The model under review builds one solid part; all positions refer to its coordinate system, in mm. A direction names the side the tool comes from. Coordinates: 2 decimals unless noted, no trailing zeros. Write each loop counter-clockwise with the first axis right and the second up, starting at its lowest first coordinate (ties: lowest second). Pieces come first, ordered by that corner, then holes.
1) Add section C-C, the plane x = 2.5. State the section outline as (y, z) points.
2) Add section B-B, the plane z = 40. State the section outline as (x, y) points.
3) For P1, Ø0.6, axis at y = -29.5, z = 53.5, coming from the +X side; P2, Ø10, axis at y = 19, z = 23.5, coming from the +X side; P3, Ø0.6, axis at x = 7, z = 53.5, coming from the +Y side, all flat-tipped, find the tip position at first contact; note any pin that passes through.
4) Mouldability with a two-part tool opening along Y and no side actions: class faces 1 (the cylindrical face through (27.3, 0.2, 77.5)), 2 (the flat face through (-6.705, 9, 45)), 3 (the cylindrical face through (41, -29, 73)), 4 (the flat face through (19.34, -34, 40)) as released by +Y, released by -Y, zero draft, split by the parting line, or undercut.
5) Add section A-A, the plane y = 0. State the section outline as (x, z) points, then the cut area to 3 significant figures.
6) Machinability: for faces 5 (the flat face through (6, -30, 67)), 6 (the flat face through (34.9, -28, 53.3)), 7 (the cylindrical face through (-7.21, 2.6, 59.83)), 8 (the flat face through (34, -34, 27)), 9 (the flat face through (-4, 40, 43)), which of the approach directions +Z, -Z, +X, -X, +Y, -Y give a long, thin tool a straight path to every point of the face, cutting with its end or side? Answer none if there is none.
7) For line 1 (Z direction, x = -4.7, y = 0); line 2 (Z direction, x = 29.5, y = 25); line 3 (X direction, y = 10.5, z = 14), list the stretches that pass through material, from the lowest coordinate up.
from build123d import *

# Parameters (mm, degrees)
SKETCH1_R           = 4.9999999999999964
BOSS_EXTRUDE1_DEPTH = 5
BOSS_EXTRUDE2_DEPTH = 70
BOSS_EXTRUDE3_DEPTH = 70
CUT_EXTRUDE1_DEPTH  = 5
SKETCH6_R           = 20.000000000000004
CUT_EXTRUDE2_DEPTH  = 1
CUT_EXTRUDE3_DEPTH  = 19.000000000000004
BOSS_EXTRUDE4_DEPTH = 1.9999999999999896
FILLET1_R           = 5
CUT_EXTRUDE4_DEPTH  = 27.00000000000001
BOSS_EXTRUDE5_DEPTH = 2
BOSS_EXTRUDE6_DEPTH = 2


with BuildPart() as part:
    # Sketch1 → Boss-Extrude1 (new body)
    with BuildSketch(Plane.XY):
        with BuildLine():
            Line((-7.704615384615421, -40.00000000000001), (32.295384615384584, -40.00000000000001))
            ThreePointArc((32.295384615384584, -40.00000000000001), (72.29538461538459, 0), (32.29538461538458, 39.99999999999999))
            Line((32.29538461538458, 39.99999999999999), (-7.7046153846154315, 39.99999999999999))
            Line((-7.7046153846154315, 39.99999999999999), (-7.704615384615421, -40.00000000000001))
        make_face()
        with Locations((32.295384615384584, 0)):
            Circle(SKETCH1_R, mode=Mode.SUBTRACT)
    boss_extrude1 = extrude(amount=BOSS_EXTRUDE1_DEPTH)

    # Sketch2 → Boss-Extrude2 (add)
    with BuildSketch(Plane.XY.offset(5)):
        Polygon((-7.7046153846154315, 39.99999999999999), (-2.70461538461543, 39.99999999999999), (-2.7046153846154235, -40.00000000000001), (-7.704615384615421, -40.00000000000001), align=None)
    extrude(amount=BOSS_EXTRUDE2_DEPTH)

    # Mirror1: Boss-Extrude1 across plane
    add(boss_extrude1.mirror(Plane.XY.offset(40)))

    # Sketch4 → Boss-Extrude3 (add)
    with BuildSketch(Plane.XY.offset(5)):
        with BuildLine():
            Line((-2.7046153846154266, -40.00000000000001), (-2.7046153846154266, -30.000000000000007))
            Line((-2.7046153846154266, -30.000000000000007), (43.497251593214216, -30.000000000000007))
            Line((43.497251593214216, -30.000000000000007), (58.7528977260305, -30.000000000000007))
            ThreePointArc((58.7528977260305, -30.000000000000007), (46.43752023911554, -37.41657386773942), (32.295384615384584, -40.00000000000001))
            Line((32.295384615384584, -40.00000000000001), (-2.7046153846154266, -40.00000000000001))
        make_face()
    extrude(amount=BOSS_EXTRUDE3_DEPTH)

    # Sketch5 → Cut-Extrude1 (cut)
    with BuildSketch(Plane.ZY.offset(7.704615384615426)):
        with BuildLine():
            ThreePointArc((50.00000000000001, -1.388e-14), (43.82683432365097, 9.238795325112829), (32.92893218813463, 7.071067811865561))
            Line((32.92893218813452, 7.0710678118654755), (47.071067811865476, -7.071067811865483))
            ThreePointArc((47.0710678118656, -7.0710678118653725), (49.2387953251129, -3.826834323650836), (50.00000000000001, -1.633e-14))
        make_face()
        with BuildLine():
            Line((47.071067811865476, -7.071067811865483), (32.92893218813452, 7.0710678118654755))
            ThreePointArc((32.92893218813463, 7.071067811865561), (32.92893218813454, -7.071067811865502), (47.0710678118656, -7.0710678118653725))
        make_face()
    extrude(amount=-CUT_EXTRUDE1_DEPTH, mode=Mode.SUBTRACT)

    # Sketch6 → Cut-Extrude2 (cut)
    with BuildSketch(Plane.ZY.offset(7.704615384615426)):
        with Locations(Location((40.00000000000001, -1.388e-14, 0), (0, 0, 270))):
            Circle(SKETCH6_R)
    extrude(amount=-CUT_EXTRUDE2_DEPTH, mode=Mode.SUBTRACT)

    # Sketch7 → Cut-Extrude3 (cut)
    with BuildSketch(Plane(origin=(0, -30.000000000000007, 0), x_dir=(1, 0, 0), z_dir=(0, 1, 0))):
        Polygon((58.7528977260305, -53.00000000000001), (58.7528977260305, -40.00000000000001), (58.7528977260305, -27.000000000000004), (19.339689979409883, -27.000000000000007), (19.339689979409883, -53.00000000000001), align=None)
    extrude(amount=-CUT_EXTRUDE3_DEPTH, mode=Mode.SUBTRACT)

    # Sketch8 → Boss-Extrude4 (add)
    with BuildSketch(Plane(origin=(0, -30.000000000000007, 0), x_dir=(1, 0, 0), z_dir=(0, 1, 0))):
        Polygon((58.7528977260305, -53.00000000000001), (19.33968997940988, -53.00000000000001), (19.33968997940988, -27.000000000000007), (58.7528977260305, -27.000000000000004), (58.7528977260305, -25.000000000000007), (56.7528977260305, -25.000000000000007), (17.33968997940988, -25.000000000000007), (17.33968997940988, -55.00000000000001), (58.7528977260305, -55.00000000000001), align=None)
    extrude(amount=BOSS_EXTRUDE4_DEPTH)

    # Fillet1
    fillet1_edges = [part.edges().sort_by_distance(p)[0] for p in [
        (-7.704615384615421, -40.00000000000001, 40),
        (28.024141170707534, -30.000000000000007, 5),
        (28.024141170707537, -30.000000000000007, 75),
    ]]
    fillet(fillet1_edges, radius=FILLET1_R)

    # Sketch9 → Cut-Extrude4 (cut)
    with BuildSketch(Plane(origin=(0, -30.000000000000007, 0), x_dir=(1, 0, 0), z_dir=(0, 1, 0))):
        Polygon((-2.7046153846154266, -69.99999999999999), (-2.70461538461543, -5), (17.295384615384563, -5), (17.295384615384574, -75), (-2.7046153846154266, -75), align=None)
    extrude(amount=CUT_EXTRUDE4_DEPTH, mode=Mode.SUBTRACT)

    # Sketch10 → Boss-Extrude5 (add)
    with BuildSketch(Plane(origin=(0, -30.000000000000007, 0), x_dir=(1, 0, 0), z_dir=(0, 1, 0))):
        Polygon((15.795384615384572, -52.5), (13.795384615384577, -52.5), (-2.704615384615426, -52.5), (-2.7046153846154257, -54.5), (15.79538461538457, -54.5), align=None)
    extrude(amount=BOSS_EXTRUDE5_DEPTH)

    # Sketch11 → Boss-Extrude6 (add)
    with BuildSketch(Plane(origin=(0, -30.000000000000007, 0), x_dir=(1, 0, 0), z_dir=(0, 1, 0))):
        Polygon((-2.704615384615427, -56.849999999999994), (-2.7046153846154266, -58.24999999999999), (15.895384615384575, -58.24999999999999), (15.895384615384579, -75), (17.295384615384574, -75), (17.295384615384574, -69.99999999999999), (17.295384615384574, -56.849999999999994), align=None)
    extrude(amount=BOSS_EXTRUDE6_DEPTH)


solid = part.part
Geometry results:
1. outline: (-40, 0) - (40, 0) - (40, 5) - (-30, 5) - (-30, 52.5) - (-28, 52.5) - (-28, 54.5) - (-30, 54.5) - (-30, 56.85) - (-28, 56.85) - (-28, 58.25) - (-30, 58.25) - (-30, 75) - (40, 75) - (40, 80) - (-40, 80) - close
2. outline: (-7.7, -35) arc R5 ccw to (-2.7, -40) - (19.34, -40) - (19.34, -28) - (17.34, -28) - (17.34, -30) - (-2.7, -30) - (-2.7, -10) - (-6.7, -10) - (-6.7, -20) - (-7.7, -20) - close; (-7.7, 20) - (-6.7, 20) - (-6.7, 10) - (-2.7, 10) - (-2.7, 40) - (-7.7, 40) - close
3. P1: stops at x = 58.75
3. P2: stops at x = -2.7
3. P3: stops at y = -28
4. face 1: undercut
4. face 2: undercut
4. face 3: released by +Y
4. face 4: zero draft
5. outline: (-7.7, 0) - (27.3, 0) - (27.3, 5) - (-2.7, 5) - (-2.7, 30) - (-6.7, 30) - (-6.7, 20) - (-7.7, 20) - close; (-7.7, 60) - (-6.7, 60) - (-6.7, 50) - (-2.7, 50) - (-2.7, 75) - (27.3, 75) - (27.3, 80) - (-7.7, 80) - close; (37.3, 0) - (72.3, 0) - (72.3, 5) - (37.3, 5) - close; (37.3, 75) - (72.3, 75) - (72.3, 80) - (37.3, 80) - close
5. area: 930 mm2
6. face 5: +Y
6. face 6: +X, +Y
6. face 7: -X
6. face 8: +X, +Y, -Y
6. face 9: +Z, -Z, +X, -X, +Y
7. line 1: z = 0 to 30, 50 to 80
7. line 2: z = 0 to 5, 75 to 80
7. line 3: x = -7.7 to -2.7
